Check sheet for the modelled part. Datum: model origin and axes. Units: mm. Round coordinates to 2 decimals unless told otherwise and drop trailing zeros. Order: outer loops, then holes, each group sorted by start corner. A loop starts at its lowest first (then second) coordinate and runs counter-clockwise, first axis right, second up.
```python
from build123d import *

# Parameters (mm, degrees)
SKETCH1_W           = 498.348
SKETCH1_H           = 165.1
BOSS_EXTRUDE1_DEPTH = 1.143
SKETCH2_W           = 69.85
SKETCH2_H           = 2.286
BOSS_EXTRUDE2_DEPTH = 3.175
LPATTERN1_COUNT     = 5
LPATTERN1_PITCH     = 98.8568
SKETCH3_R           = 5
CUT_EXTRUDE1_DEPTH  = 264.517900145


with BuildPart() as part:
    # Sketch1 → Boss-Extrude1 (new, symmetric)
    with BuildSketch(Plane(origin=(0, 0, 0), x_dir=(1, 0, 0), z_dir=(0, 1, 0))):
        Rectangle(SKETCH1_W, SKETCH1_H)
    extrude(amount=BOSS_EXTRUDE1_DEPTH, both=True)

    # Sketch2 → Boss-Extrude2 (add)
    with BuildSketch(Plane(origin=(0, 0, -82.55), x_dir=(-1, 0, 0), z_dir=(0, 0, -1))):
        with Locations((-197.7136, 0)):
            Rectangle(SKETCH2_W, SKETCH2_H)
    boss_extrude2 = extrude(amount=BOSS_EXTRUDE2_DEPTH)

    # LPattern1: Boss-Extrude2 ×5
    with Locations(*[(-i * LPATTERN1_PITCH, 0, 0) for i in range(1, LPATTERN1_COUNT)]):
        add(boss_extrude2)

    # Sketch3 → Cut-Extrude1 (cut, through all)
    with BuildSketch(Plane.XZ.offset(1.143)):
        with Locations(Location((-155.3337, 3.9751, 0), (0, 0, 270))):
            Circle(SKETCH3_R)
        with Locations(Location((-141.2367, 3.9751, 0), (0, 0, 270))):
            Circle(SKETCH3_R)
        with Locations(Location((-141.2367, -8.7249, 0), (0, 0, 270))):
            Circle(SKETCH3_R)
        with Locations(Location((-155.3337, -8.7249, 0), (0, 0, 270))):
            Circle(SKETCH3_R)
        with Locations(Location((-141.2367, -21.4249, 0), (0, 0, 270))):
            Circle(SKETCH3_R)
        with Locations(Location((-155.3337, -21.4249, 0), (0, 0, 270))):
            Circle(SKETCH3_R)
        with Locations(Location((-141.2367, -34.1249, 0), (0, 0, 270))):
            Circle(SKETCH3_R)
        with Locations(Location((-155.3337, -34.1249, 0), (0, 0, 270))):
            Circle(SKETCH3_R)
        with Locations(Location((56.4769, 3.9751, 0), (0, 0, 270))):
            Circle(SKETCH3_R)
        with Locations(Location((56.4769, -8.7249, 0), (0, 0, 270))):
            Circle(SKETCH3_R)
        with Locations(Location((42.3799, 3.9751, 0), (0, 0, 270))):
            Circle(SKETCH3_R)
        with Locations(Location((42.3799, -8.7249, 0), (0, 0, 270))):
            Circle(SKETCH3_R)
        with Locations(Location((56.4769, -21.4249, 0), (0, 0, 270))):
            Circle(SKETCH3_R)
        with Locations(Location((42.3799, -21.4249, 0), (0, 0, 270))):
            Circle(SKETCH3_R)
        with Locations(Location((56.4769, -34.1249, 0), (0, 0, 270))):
            Circle(SKETCH3_R)
        with Locations(Location((42.3799, -34.1249, 0), (0, 0, 270))):
            Circle(SKETCH3_R)
        with Locations(Location((155.3337, 3.9751, 0), (0, 0, 270))):
            Circle(SKETCH3_R)
        with Locations(Location((155.3337, -8.7249, 0), (0, 0, 270))):
            Circle(SKETCH3_R)
        with Locations(Location((155.3337, -21.4249, 0), (0, 0, 270))):
            Circle(SKETCH3_R)
        with Locations(Location((155.3337, -34.1249, 0), (0, 0, 270))):
            Circle(SKETCH3_R)
    extrude(amount=-CUT_EXTRUDE1_DEPTH, mode=Mode.SUBTRACT)


solid = part.part
```
Item 1: Sectioned sample at A-A (z = -34.5). Record the cut outline in (x, y), and give its area (3 significant figures).
Answer:
outline: (-249.17, -1.14) - (-160.32, -1.14) - (-160.32, 1.14) - (-249.17, 1.14) - close; (-150.35, -1.14) - (-146.22, -1.14) - (-146.22, 1.14) - (-150.35, 1.14) - close; (-136.25, -1.14) - (37.39, -1.14) - (37.39, 1.14) - (-136.25, 1.14) - close; (47.37, -1.14) - (51.49, -1.14) - (51.49, 1.14) - (47.37, 1.14) - close; (61.46, -1.14) - (150.35, -1.14) - (150.35, 1.14) - (61.46, 1.14) - close; (160.32, -1.14) - (249.17, -1.14) - (249.17, 1.14) - (160.32, 1.14) - close
area: 1,030 mm2
Item 2: Scan lines: line 1 along Z through (x, y) = (-144, -0.65); line 2 along X through (y, z) = (0.35, -24.5); line 3 along X through (y, z) = (1, -33). Record each from-to range of solid material in increasing order.
Answer:
line 1: z = -82.55 to -38.29, -29.96 to -25.59, -17.26 to -12.89, -4.56 to -0.19, 8.14 to 82.55
line 2: x = -249.17 to -159.28, -151.39 to -145.18, -137.29 to 38.44, 46.32 to 52.53, 60.42 to 151.39, 159.28 to 249.17
line 3: x = -249.17 to -160.21, -150.46 to -146.11, -136.36 to 37.51, 47.25 to 51.61, 61.35 to 150.46, 160.21 to 249.17
Item 3: Go/stop test with a flat-tipped pin: P1, Ø0.7, axis at y = 0.5, z = -84.5, coming from the +X side. Record where the tip stops, or that it passes through.
Answer:
P1: stops at x = 232.64
Item 4: Sectioned sample at B-B (y = 0.4). State how many separate pieces and enclosed holes the cut face has, and give its area (3 significant figures).
Answer:
separate pieces: 1
enclosed holes: 20
area: 81,800 mm2
Item 5: Release check for a two-part mould opening along X. For faces 1 (the cylindrical face through (39.337, -0.016, 7.943)), 2 (the flat face through (-3, -1.143, -3)) record: released by +X, released by -X, zero draft, split by the parting line, or undercut.
Answer:
face 1: undercut
face 2: zero draft
